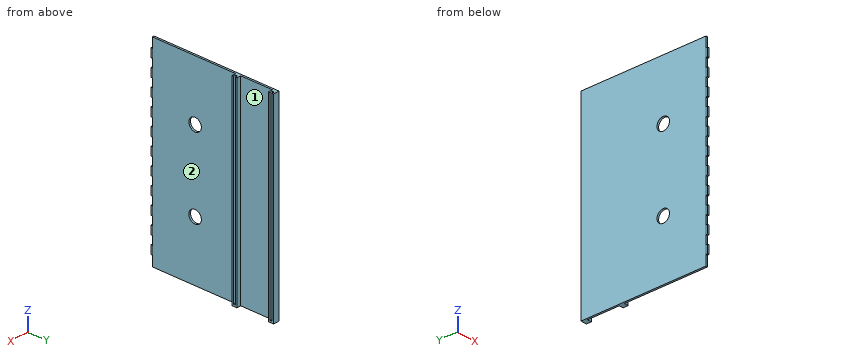
from build123d import *

# Parameters (mm, degrees)
SKETCH_4_W          = 233.6
SKETCH_4_H          = 150
EXTRUDE_2_DEPTH     = 2.2
SKETCH_6_W          = 2
SKETCH_6_H          = 10
EXTRUDE_3_DEPTH     = 1.8
SKETCH_7_W          = 233.6
SKETCH_7_H          = 6
EXTRUDE_4_DEPTH     = 5
SKETCH_8_W          = 114.8
SKETCH_8_H          = 2.2
SKETCH_8_W_2        = 116.8
SKETCH_8_W_3        = 231.6
CUT_EXTRUDE_1_DEPTH = 3
SKETCH1_R           = 7.5
CUT_EXTRUDE1_DEPTH  = 10


with BuildPart() as part:
    # 草图4 → 凸台-拉伸2 (new body)
    with BuildSketch(Plane(origin=(0, 0, 0), x_dir=(0, 0, -1), z_dir=(1, 0, 0))):
        Rectangle(SKETCH_4_W, SKETCH_4_H)
    extrude(amount=EXTRUDE_2_DEPTH)

    # 草图6 → 凸台-拉伸3 (add)
    with BuildSketch(Plane.XZ.offset(75)):
        with Locations((1.1, 20)):
            Rectangle(SKETCH_6_W, SKETCH_6_H)
        with Locations((1.1, 0)):
            Rectangle(SKETCH_6_W, SKETCH_6_H)
        with Locations((1.1, 40)):
            Rectangle(SKETCH_6_W, SKETCH_6_H)
        with Locations((1.1, 60)):
            Rectangle(SKETCH_6_W, SKETCH_6_H)
        with Locations((1.1, 80)):
            Rectangle(SKETCH_6_W, SKETCH_6_H)
        with Locations((1.1, 100)):
            Rectangle(SKETCH_6_W, SKETCH_6_H)
        with Locations((1.1, -20)):
            Rectangle(SKETCH_6_W, SKETCH_6_H)
        with Locations((1.1, -40)):
            Rectangle(SKETCH_6_W, SKETCH_6_H)
        with Locations((1.1, -60)):
            Rectangle(SKETCH_6_W, SKETCH_6_H)
        with Locations((1.1, -80)):
            Rectangle(SKETCH_6_W, SKETCH_6_H)
        with Locations((1.1, -100)):
            Rectangle(SKETCH_6_W, SKETCH_6_H)
    extrude(amount=EXTRUDE_3_DEPTH)

    # 草图7 → 凸台-拉伸4 (add)
    with BuildSketch(Plane(origin=(2.2, 0, 0), x_dir=(0, 0, -1), z_dir=(1, 0, 0))):
        with Locations((0, 28)):
            Rectangle(SKETCH_7_W, SKETCH_7_H)
        with Locations((0, 72)):
            Rectangle(SKETCH_7_W, SKETCH_7_H)
    extrude(amount=EXTRUDE_4_DEPTH)

    # 草图8 → 切除-拉伸1 (cut)
    with BuildSketch(Plane(origin=(7.2, 0, 0), x_dir=(0, 0, -1), z_dir=(1, 0, 0))):
        with Locations((57.4, 28)):
            Rectangle(SKETCH_8_W, SKETCH_8_H)
        with Locations((-58.4, 28)):
            Rectangle(SKETCH_8_W_2, SKETCH_8_H)
        with Locations((-1, 72)):
            Rectangle(SKETCH_8_W_3, SKETCH_8_H)
    extrude(amount=-CUT_EXTRUDE_1_DEPTH, mode=Mode.SUBTRACT)

    # Sketch1 → Cut-Extrude1 (cut)
    with BuildSketch(Plane(origin=(2.2, 0, 0), x_dir=(0, 0, -1), z_dir=(1, 0, 0))):
        with Locations((-46.8, -23.745319948)):
            Circle(SKETCH1_R)
        with Locations((46.8, -23.745319948)):
            Circle(SKETCH1_R)
    extrude(amount=-CUT_EXTRUDE1_DEPTH, mode=Mode.SUBTRACT)


solid = part.part
Work out the finished part from the listing and answer in its coordinate system (mm). Face numbers are marked on the shaded views. Coordinates: 2 decimals unless noted, no trailing zeros. Loops run counter-clockwise (first coordinate to the right, second up) from the corner with the lowest first, then second, coordinate; pieces in that order, holes last. Notation, with made-up numbers: M 57,-40 L 82,-40 A5 cw 82,-35 Z; hole C 74.5,-23.75 d3. An arc over 180 degrees is marked long. Answer in a Markdown table with one row per item. Add a question column.
1. Consider L1, parallel to Y at x = 5, z = -34; L2, parallel to Y at x = 1.4, z = -46.8; L3, parallel to Y at x = 2.5, z = 35. Determine where each line is inside the solid, lowest interval first.
2. Find section A-A, the plane x = 5.75. Write down the section's boundary in (y, z).
3. Flat-ended cylindrical pins translate along their axes: P1, Ø0.9, axis at x = 1, y = -76.5, coming from the -Z side; P2, Ø1, axis at y = -11, z = -91, coming from the +X side; P3, Ø2, axis at x = 6, z = 89.5, coming from the -Y side. Find the tip coordinate at first contact, or state that the pin passes through.
4. Find section B-B, the plane z = -48. Write down the section's boundary in (x, y), then the cut area to 3 significant figures.
5. Find section D-D, the plane y = -62. Write down the section's boundary in (x, z).
6. Find section C-C, the plane z = 7.5. Write down the section's boundary in (x, y), then the cut area to 3 significant figures.
7. The mould has two halves that part along Y. Classify the marked faces 1 and 2: pulls with the +Y half, pulls with the -Y half, needs draft (parallel to the pull), parting line crosses it, or undercut.
Reported:
| question | item | result |
|---|---|---|
| 1 | L1 | y = 25 to 26.9, 29.1 to 31, 69 to 70.9, 73.1 to 75 |
| 1 | L2 | y = -75 to -31.25, -16.25 to 75 |
| 1 | L3 | y = 25 to 31, 69 to 75 |
| 2 | outline | M 25,-116.8 L 31,-116.8 L 31,116.8 L 29.1,116.8 L 29.1,-114.8 L 26.9,-114.8 L 26.9,116.8 L 25,116.8 Z; M 69,-116.8 L 75,-116.8 L 75,116.8 L 73.1,116.8 L 73.1,-114.8 L 70.9,-114.8 L 70.9,116.8 L 69,116.8 Z |
| 3 | P1 | stops at z = -105 |
| 3 | P2 | stops at x = 2.2 |
| 3 | P3 | stops at y = 25 |
| 4 | outline | M 0,-75 L 2.2,-75 L 2.2,-31.15 L 0,-31.15 Z; M 0,-16.34 L 2.2,-16.34 L 2.2,25 L 7.2,25 L 7.2,26.9 L 4.2,26.9 L 4.2,29.1 L 7.2,29.1 L 7.2,31 L 2.2,31 L 2.2,69 L 7.2,69 L 7.2,70.9 L 4.2,70.9 L 4.2,73.1 L 7.2,73.1 L 7.2,75 L 0,75 Z |
| 4 | area | 344 mm^2 |
| 5 | outline | M 0,-116.8 L 2.2,-116.8 L 2.2,116.8 L 0,116.8 Z |
| 6 | outline | M 0,-75 L 2.2,-75 L 2.2,25 L 7.2,25 L 7.2,26.9 L 4.2,26.9 L 4.2,29.1 L 7.2,29.1 L 7.2,31 L 2.2,31 L 2.2,69 L 7.2,69 L 7.2,70.9 L 4.2,70.9 L 4.2,73.1 L 7.2,73.1 L 7.2,75 L 0,75 Z |
| 6 | area | 377 mm^2 |
| 7 | face 1 | undercut |
| 7 | face 2 | needs draft |
